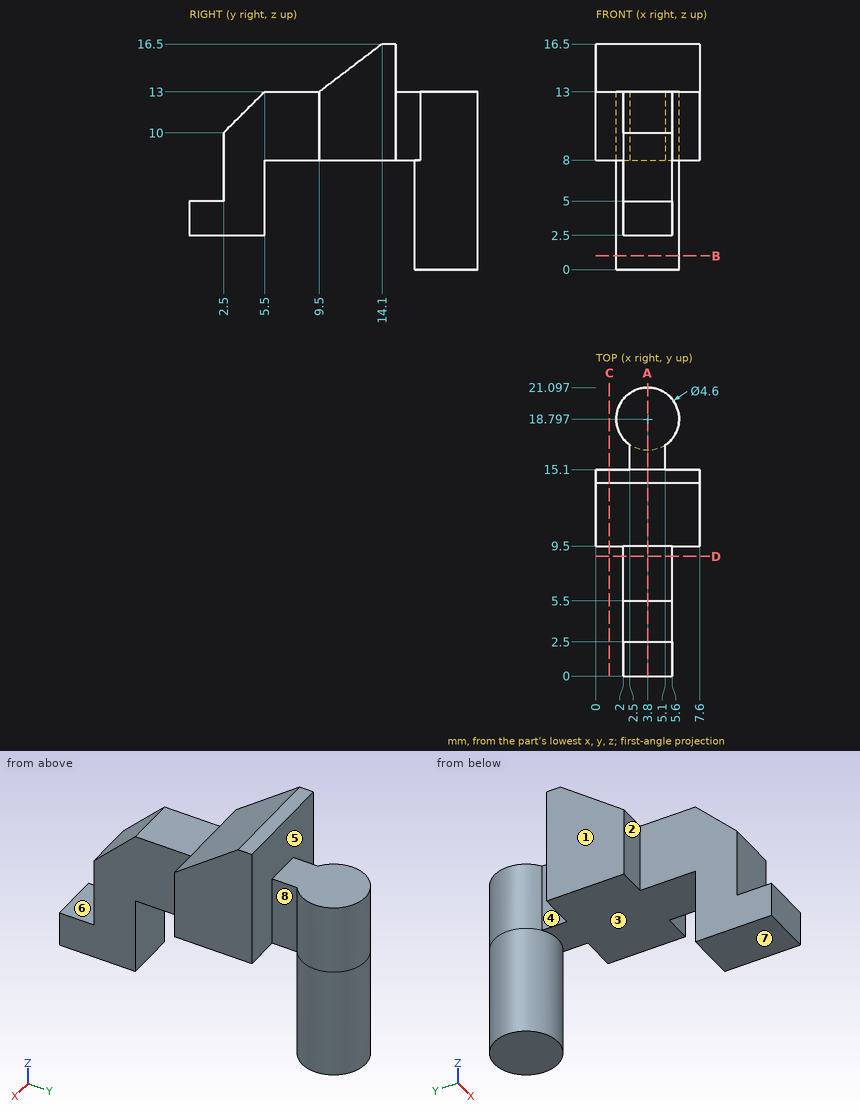
Job drawing, mm, ordinate dimensions from the low corner. One solid piece. A direction names the side the tool comes from. Coordinates: 2 decimals unless noted, no trailing zeros. Loops run counter-clockwise (first coordinate to the right, second up) from the corner with the lowest first, then second, coordinate; pieces in that order, holes last. Notation, with made-up numbers: (-38.5, 69.5) - (-27.5, 69.5) arc R19 cw to (-27.5, 75.5) - close; hole circle Ø7 at (-15, 56.5). An arc over 180 degrees is marked (long way). Write item = value, one per line. Start each with the question number.
Q1. Pull direction Y, two halves, no side cores. Call the marked faces 1, 2, 3 and 4: pulls with the +Y half, pulls with the -Y half, needs draft (parallel to the pull), parting line crosses it, or undercut.
Q2. Cut at A-A, the plane x = 3.8. List the corners of the cut face in (y, z), then the cut area to 3 significant figures.
Q3. Drill centre lines: L1, parallel to X at y = 15.75, z = 11; L2, parallel to Y at x = 4.5, z = 3.5; L3, parallel to Z at x = 4.5, y = 15. Where is each one in solid material? Low to high.
Q4. Cut at B-B, the plane z = 1. List the corners of the cut face in (x, y), then the cut area to 3 significant figures.
Q5. Cut at C-C, the plane x = 1. List the corners of the cut face in (y, z).
Q6. Which spindle directions (+Z, -Z, +X, -X, +Y, -Y) get a long thin tool onto all of the face, cutting with end or side? Do the marked faces 5, 6, 7 and 8. Say none if no direction does.
Q7. Flat gauge pins, fed straight in: pin 1 Ø2 at (y, z) = (18.5, 7.5) entering from +X; pin 2 Ø8 at (y, z) = (4.5, 8.5) entering from +X; pin 3 Ø1.5 at (y, z) = (16.5, 8) entering from -X. Where does each tip first touch, or does it go through?
Q8. Cut at D-D, the plane y = 8.75. List the corners of the cut face in (x, z).
Computed:
q1.face_1 = needs draft
q1.face_2 = pulls with the -Y half
q1.face_3 = undercut
q1.face_4 = undercut
q2.outline = (0, 2.5) - (5.5, 2.5) - (5.5, 8) - (16.5, 8) - (16.5, 0) - (21.1, 0) - (21.1, 13) - (15.1, 13) - (15.1, 16.5) - (14.1, 16.5) - (9.5, 13) - (5.5, 13) - (2.5, 10) - (2.5, 5) - (0, 5) - close
q2.area = 160 mm²
q3.L1 = 2.5 to 5.1
q3.L2 = 0 to 5.5, 16.61 to 20.99
q3.L3 = 8 to 16.5
q4.outline = circle Ø4.6 at (3.8, 18.8)
q4.area = 16.6 mm²
q5.outline = (9.5, 8) - (15.1, 8) - (15.1, 16.5) - (14.1, 16.5) - (9.5, 13) - close
q6.face_5 = +Z
q6.face_6 = +Z, +X, -X, -Y
q6.face_7 = -Z, +X, -X, -Y
q6.face_8 = +Z, -Z, +X
q7.pin_1 = 6.1
q7.pin_2 = 5.6
q7.pin_3 = 2.1
q8.outline = (2, 8) - (5.6, 8) - (5.6, 13) - (2, 13) - close
